Geometry check sheet. Reference: the model listing, model coordinates, mm. Face numbers are marked on the shaded views. Coordinates: 2 decimals unless noted, no trailing zeros. Loops run counter-clockwise (first coordinate to the right, second up) from the corner with the lowest first, then second, coordinate; pieces in that order, holes last. Notation, with made-up numbers: (-1, 51.25) -> (35, 51.25) arc R13 cw to (35, 66.25) -> close; hole circle Ø6 at (-40, 8.25). An arc over 180 degrees is marked (long way). Answer as a JSON object with one key per item and string values.
from build123d import *

# Parameters (mm, degrees)
BOSS_EXTRUDE1_START = -3
SKETCH1_R           = 3.3
BOSS_EXTRUDE1_DEPTH = 1


with BuildPart() as part:
    # Sketch1 → Boss-Extrude1 (new body)
    with BuildSketch(Plane.XY.offset(BOSS_EXTRUDE1_START)):
        with BuildLine():
            Line((175.530545653, 297.078241002), (165.847660098, 286.247140349))
            add(Edge.make_bspline(
                [(165.847660098, 286.247140349), (161.958951275, 288.053215105), (153.7541863, 291.385632032), (142.949710049, 287.922349017), (132.08866755, 288.696875058), (123.730011038, 286.762274271), (122.229813512, 281.878394702)],
                knots=[0, 0, 0, 0, 0.282569956, 0.534959137, 0.697744118, 1, 1, 1, 1], degree=3))
            add(Edge.make_bspline(
                [(122.229813512, 281.878394702), (118.058976155, 279.823016138), (111.235657544, 270.739838071), (106.106560937, 260.813884877), (101.703831056, 255.636584821)],
                knots=[0, 0, 0, 0, 0.398895915, 1, 1, 1, 1], degree=3))
            add(Edge.make_bspline(
                [(101.703831056, 255.636584821), (100.938919323, 251.235797266), (103.183355148, 242.927772517), (104.33056652, 234.543938083), (106.075647572, 230.779395719)],
                knots=[0, 0, 0, 0, 0.517213565, 1, 1, 1, 1], degree=3))
            add(Edge.make_bspline(
                [(106.075647572, 230.779395719), (103.798133299, 224.247937083), (105.543362439, 217.548369999)],
                knots=[0, 0, 0, 1, 1, 1], degree=2))
            add(Edge.make_bspline(
                [(105.543362439, 217.548369999), (101.478949421, 216.275176704), (89.438329667, 214.004143017), (82.364872068, 202.984357934), (75.608431069, 199.787338704)],
                knots=[0, 0, 0, 0, 0.364395461, 1, 1, 1, 1], degree=3))
            add(Edge.make_bspline(
                [(75.608431069, 199.787338704), (72.965008377, 200.448410696), (68.130105896, 201.670017191), (62.019757504, 202.966820343), (54.835011624, 201.049857451), (56.921255323, 196.431484587), (58.321643082, 193.17869111), (58.082321369, 189.161546227), (61.757389476, 184.075704484), (65.851558074, 182.053410846), (67.551159033, 179.262120633)],
                knots=[0, 0, 0, 0, 0.185122606, 0.320265005, 0.454108381, 0.537288926, 0.599177691, 0.700070158, 0.790196975, 1, 1, 1, 1], degree=3))
            add(Edge.make_bspline(
                [(67.551159033, 179.262120633), (63.651335521, 175.669295098), (59.980616164, 171.840128471)],
                knots=[0, 0, 0, 1, 1, 1], degree=2))
            add(Edge.make_bspline(
                [(59.980616164, 171.840128471), (58.13524604, 170.76965569), (56.3909212, 168.715252622), (56.887266336, 166.42033094)],
                knots=[0, 0, 0, 0, 1, 1, 1, 1], degree=3))
            ThreePointArc((56.887266336, 166.42033094), (56.001787201, 164.093208994), (55.156159125, 161.751311683))
            Line((55.156159125, 161.751311683), (16.490969335, 118.53562592))
            ThreePointArc((16.490969335, 118.53562592), (13.594458931, 116.03119733), (10.158239499, 114.341720756))
            ThreePointArc((10.158239499, 114.341720756), (7.138291038, 109.59789587), (11.104930852, 105.61170322))
            ThreePointArc((11.104930852, 105.61170322), (14.823431664, 104.698091272), (18.189463296, 102.87277866))
            Line((18.189463296, 102.87277866), (158.308378587, 1.805164583))
            ThreePointArc((158.308378587, 1.805164583), (161.577939242, 0.872224158), (164.688165503, 2.245867969))
            Line((164.688165503, 2.245867969), (276.957680669, 109.555734945))
            ThreePointArc((276.957680669, 109.555734945), (280.040760403, 111.826539744), (283.598320347, 113.242767948))
            ThreePointArc((283.598320347, 113.242767948), (286.933122885, 116.94588976), (284.808210365, 121.45352394))
            ThreePointArc((284.808210365, 121.45352394), (281.810364375, 123.835719251), (279.51333018, 126.899306851))
            Line((279.51333018, 126.899306851), (183.60866827, 296.210136052))
            ThreePointArc((183.60866827, 296.210136052), (179.792379546, 298.717191637), (175.530545653, 297.078241002))
        make_face()
        with Locations((11.612063393, 110.083035973)):
            Circle(SKETCH1_R, mode=Mode.SUBTRACT)
        with Locations((282.4811963, 117.601900186)):
            Circle(SKETCH1_R, mode=Mode.SUBTRACT)
    extrude(amount=-BOSS_EXTRUDE1_DEPTH)


solid = part.part
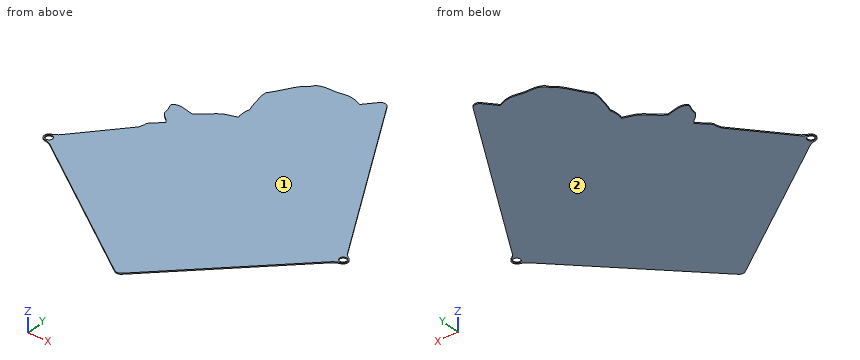
1. Section check A-A, the plane y = 80. Record the boundary of the cut face in (x, z).
Evaluation:
{"outline": "(49.9, -4) -> (246.04, -4) -> (246.04, -3) -> (49.9, -3) -> close"}
2. Mould release check, pull along Z, two halves, no side actions. Record for the marked faces 1 and 2: released by +Z, released by -Z, zero draft, split by the parting line, or undercut.
Evaluation:
{"face 1": "released by +Z", "face 2": "released by -Z"}
3. Section check C-C, the plane z = -3.6. State how many separate pieces and enclosed holes the cut face has, then the cut area to 3 significant figures.
Evaluation:
{"separate pieces": "1", "enclosed holes": "2", "area": "44,400 mm^2"}
4. Section check B-B, the plane x = 203.5. Record the boundary of the cut face in (y, z), then the cut area to 3 significant figures.
Evaluation:
{"outline": "(39.34, -4) -> (261.09, -4) -> (261.09, -3) -> (39.34, -3) -> close", "area": "222 mm^2"}
5. Depth check by flat-ended pin: P1, Ø5.5, axis at x = 11.61, y = 110.08, coming from the -Z side. Enter the tip coordinate at first touch or a pass-through.
Evaluation:
{"P1": "passes through"}
6. Thickness scan on probe 1 along Y at (x, z) = (60, -3.3); probe 2 along Y at (x, z) = (122, -3.1); probe 3 along Y at (x, z) = (256, -3.2). Record the ranges inside material, lowest first. Write a range as from..to.
Evaluation:
{"probe 1": "y = 72.71..171.86, 186.64..202.21", "probe 2": "y = 27.99..281.76", "probe 3": "y = 89.52..168.41"}
